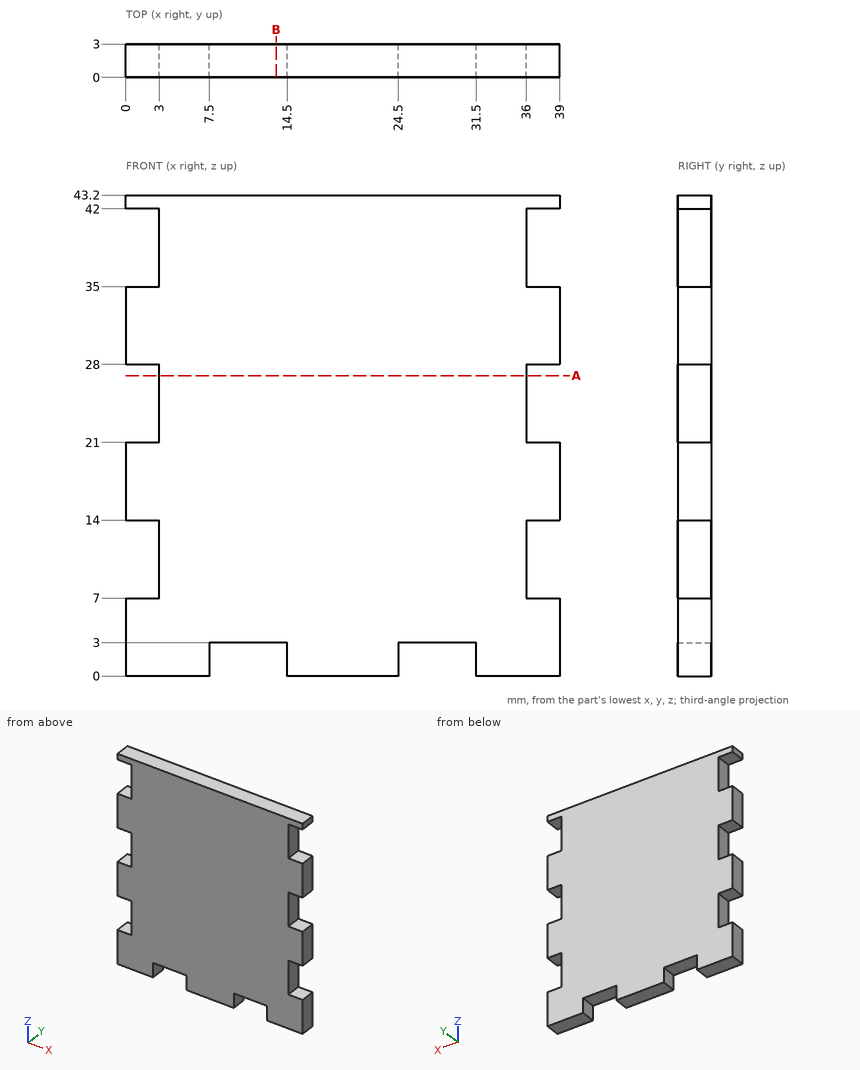
Design review of the part shown in the three views and the two pictorial views. Dimensions are in mm from the part's minimum x, y and z. Round coordinates to 2 decimals unless told otherwise and drop trailing zeros. Loops run counter-clockwise (first coordinate to the right, second up) from the corner with the lowest first, then second, coordinate; pieces in that order, holes last. Notation, with made-up numbers: (23, 84) -> (43, 84) arc R25 cw to (43, 112) -> close; hole circle Ø9 at (24.5, -3). An arc over 180 degrees is marked (long way). Answer as a JSON object with one key per item and string values. Group by question number.
1) We need section B-B on x = 13.5. Write out the cut boundary in (y, z), then the cut area to 3 significant figures.
2) We need section A-A on z = 27. Write out the cut boundary in (x, y).
3) For line 1 (Z direction, x = 9, y = 2.75); line 2 (X direction, y = 2.45, z = 13.5), list the stretches that pass through material, from the lowest coordinate up. Write a range as [from, to].
4) For pin 1 Ø1.5 at (x, z) = (25.5, 33.5) entering from -Y; pin 2 Ø1.5 at (x, y) = (11.5, 1.5) entering from -Z, all flat-tipped, find the tip position at first contact; note any pin that passes through.
Result set:
{
 "1": {"outline": "(0, 3) -> (3, 3) -> (3, 43.2) -> (0, 43.2) -> close", "area": "121 mm²"},
 "2": {"outline": "(3, 0) -> (36, 0) -> (36, 3) -> (3, 3) -> close"},
 "3": {"line 1": "[3, 43.2]", "line 2": "[3, 36]"},
 "4": {"pin 1": "y = 0", "pin 2": "z = 3"}
}
